Input: part model. Units: mm. Frame: model coordinates. A direction names the side the tool comes from. Coordinates: 2 decimals unless noted, no trailing zeros.
from build123d import *

# Parameters (mm, degrees)
SKETCH1_W               = 20
SKETCH1_H               = 20
SKETCH1_R               = 18.6
BOSS_EXTRUDE1_DEPTH     = 25
FILLET1_R               = 170
FILLET2_R               = 170
FILLET3_R               = 3
BOSS_EXTRUDE2_START     = -20
SKETCH2_R               = 18.6
SKETCH2_R_2             = 17.6
BOSS_EXTRUDE2_DEPTH     = 16
CHAMFER1_SIZE           = 0.5
CUT_EXTRUDE1_DEPTH      = 96
CUT_EXTRUDE1_DEPTH_BACK = 16
CUT_EXTRUDE2_START      = -8.5
SKETCH4_R               = 2.9
CUT_EXTRUDE2_DEPTH      = 46
CUT_EXTRUDE3_START      = -8
SKETCH5_R               = 1.48
CUT_EXTRUDE3_DEPTH      = 46


with BuildPart() as part:
    # Sketch1 → Boss-Extrude1 (new body)
    with BuildSketch(Plane(origin=(0, 0, 0), x_dir=(1, 0, 0), z_dir=(0, 1, 0))):
        with BuildLine():
            Line((-78.9, -20), (78.9, -20))
            Line((78.9, -20), (142.053074305, -14.2536949))
            ThreePointArc((142.053074305, -14.2536949), (167.546506822, 19.026935088), (132.290205184, 41.709717738))
            Line((132.290205184, 41.709717738), (48.9, 20))
            Line((48.9, 20), (7.809449404, 20))
            ThreePointArc((7.809449404, 20), (0, 14.05), (-7.809449404, 20))
            Line((-7.809449404, 20), (-48.9, 20))
            Line((-48.9, 20), (-132.290204174, 41.709717475))
            ThreePointArc((-132.290204174, 41.709717475), (-167.546506732, 19.026935602), (-142.053074305, -14.2536949))
            Line((-142.053074305, -14.2536949), (-78.9, -20))
        make_face()
        with Locations((-63.9, 0)):
            Rectangle(SKETCH1_W, SKETCH1_H, mode=Mode.SUBTRACT)
        with Locations((63.9, 0)):
            Rectangle(SKETCH1_W, SKETCH1_H, mode=Mode.SUBTRACT)
        with Locations(Location((139.47052489, 14.12905406, 0), (0, 0, 270))):
            Circle(SKETCH1_R, mode=Mode.SUBTRACT)
        with Locations(Location((-139.47052489, 14.12905406, 0), (0, 0, 270))):
            Circle(SKETCH1_R, mode=Mode.SUBTRACT)
    extrude(amount=BOSS_EXTRUDE1_DEPTH)

    # Fillet1
    # the kernel refuses this fillet: 170 mm, written as the material it takes off along each edge
    with BuildSketch(Plane(origin=(78.9, -19.295542523, 20), x_dir=(-1, 0, 0), z_dir=(0, 1, 0)), Plane(origin=(-78.9, -19.295542523, 20), x_dir=(-0.995885928416444, 0, -0.09061576894844221), z_dir=(0, 1, 0))) as fillet1_piece_1:
        with BuildLine():
            CenterArc((FILLET1_R * 0.045401276525, -FILLET1_R), FILLET1_R, 90, 5.199032807)
            Line((-FILLET1_R * 0.0452144924234, -FILLET1_R * 0.00411407158356), (0, 0))
            Line((0, 0), (FILLET1_R * 0.045401276525, 0))
        make_face()
    extrude(amount=63.591085046, mode=Mode.SUBTRACT)

    # Fillet2
    fillet2_edges = [part.edges().sort_by_distance(p)[0] for p in [
        (-48.9, 12.5, -20),
        (48.9, 12.5, -20),
    ]]
    fillet(fillet2_edges, radius=FILLET2_R)

    # Fillet3
    fillet3_edges = [part.edges().sort_by_distance(p)[0] for p in [
        (48.723757294, 25, -21.376513431),
        (-48.723757294, 0, -21.376513431),
        (-48.723757294, 25, -21.376513431),
        (167.546506822, 25, -19.026935088),
        (-167.546506732, 0, -19.026935602),
        (167.546506822, 0, -19.026935088),
        (-167.546506732, 25, -19.026935602),
        (114.319769009, 0, 16.777151365),
        (114.319769009, 25, 16.777151365),
        (0, 0, 20),
        (-114.319769009, 0, 16.777151365),
        (-78.892057589, 0, 19.825061948),
        (78.892057589, 0, 19.825061948),
        (0, 25, 20),
        (-114.319769009, 25, 16.777151365),
        (-78.892057589, 25, 19.825061948),
        (78.892057589, 25, 19.825061948),
        (17.471699722, 0, -20),
        (17.471699722, 25, -20),
        (101.12706922, 0, -33.596739912),
        (101.12706922, 25, -33.596739912),
        (-101.127068716, 0, -33.59673978),
        (-101.127068716, 25, -33.59673978),
        (-17.471699722, 0, -20),
        (-17.471699722, 25, -20),
        (48.723757294, 0, -21.376513431),
    ]]
    fillet(fillet3_edges, radius=FILLET3_R)

    # Sketch2 → Boss-Extrude2 (add)
    # profile 1 of 2: a face of its own
    with BuildSketch(Plane(origin=(0, 25, 0), x_dir=(1, 0, 0), z_dir=(0, 1, 0)).offset(BOSS_EXTRUDE2_START)):
        with Locations(Location((139.47052489, 14.12905406, 0), (0, 0, 270))):
            Circle(SKETCH2_R)
        with Locations(Location((139.47052489, 14.12905406, 0), (0, 0, 270))):
            Circle(SKETCH2_R_2, mode=Mode.SUBTRACT)
    # profile 2 of 2: a face of its own
    with BuildSketch(Plane(origin=(0, 25, 0), x_dir=(1, 0, 0), z_dir=(0, 1, 0)).offset(BOSS_EXTRUDE2_START)):
        with Locations(Location((-139.47052489, 14.12905406, 0), (0, 0, 270))):
            Circle(SKETCH2_R)
        with Locations(Location((-139.47052489, 14.12905406, 0), (0, 0, 270))):
            Circle(SKETCH2_R_2, mode=Mode.SUBTRACT)
    extrude(amount=BOSS_EXTRUDE2_DEPTH)

    # Chamfer1
    chamfer1_edges = [part.edges().sort_by_distance(p)[0] for p in [
        (139.47052489, 5, -31.72905406),
        (139.47052489, 21, -31.72905406),
        (-139.47052489, 5, -31.72905406),
        (-139.47052489, 21, -31.72905406),
    ]]
    chamfer(chamfer1_edges, length=CHAMFER1_SIZE)

    # Sketch3 → Cut-Extrude1 (cut, two sides: drawn at the far end of the back side and taken through both)
    with BuildSketch(Plane(origin=(0, 0, 10), x_dir=(-1, 0, 0), z_dir=(0, 0, -1)).offset(-CUT_EXTRUDE1_DEPTH_BACK)):
        with BuildLine():
            ThreePointArc((65.38, 12.5), (63.9, 13.98), (62.42, 12.5))
            Line((62.42, 12.5), (65.38, 12.5))
        make_face()
        with BuildLine():
            Line((65.38, 12.5), (62.42, 12.5))
            ThreePointArc((62.42, 12.5), (63.9, 11.02), (65.38, 12.5))
        make_face()
        with BuildLine():
            ThreePointArc((-62.42, 12.5), (-63.9, 13.98), (-65.38, 12.5))
            Line((-65.38, 12.5), (-62.42, 12.5))
        make_face()
        with BuildLine():
            Line((-62.42, 12.5), (-65.38, 12.5))
            ThreePointArc((-65.38, 12.5), (-63.9, 11.02), (-62.42, 12.5))
        make_face()
    extrude(amount=CUT_EXTRUDE1_DEPTH + CUT_EXTRUDE1_DEPTH_BACK, mode=Mode.SUBTRACT)

    # Sketch4 → Cut-Extrude2 (cut)
    with BuildSketch(Plane.XY.offset(-10).offset(CUT_EXTRUDE2_START)):
        with Locations((-63.9, 12.5)):
            Circle(SKETCH4_R)
        with Locations((63.9, 12.5)):
            Circle(SKETCH4_R)
    extrude(amount=-CUT_EXTRUDE2_DEPTH, mode=Mode.SUBTRACT)

    # Sketch5 → Cut-Extrude3 (cut)
    # profile 1 of 2: a face of its own
    with BuildSketch(Plane(origin=(0, 0, 10), x_dir=(-1, 0, 0), z_dir=(0, 0, -1)).offset(CUT_EXTRUDE3_START)):
        Polygon((65.525, 15.314582562), (62.275, 15.314582562), (60.65, 12.5), (62.275, 9.685417438), (65.525, 9.685417438), (67.15, 12.5), align=None)
        with Locations(Location((63.9, 12.5, 0), (0, 0, 180))):
            Circle(SKETCH5_R, mode=Mode.SUBTRACT)
    # profile 2 of 2: a face of its own
    with BuildSketch(Plane(origin=(0, 0, 10), x_dir=(-1, 0, 0), z_dir=(0, 0, -1)).offset(CUT_EXTRUDE3_START)):
        Polygon((-62.225, 15.401185103), (-65.575, 15.401185103), (-67.25, 12.5), (-65.575, 9.598814897), (-62.225, 9.598814897), (-60.55, 12.5), align=None)
    extrude(amount=-CUT_EXTRUDE3_DEPTH, mode=Mode.SUBTRACT)


solid = part.part
Item 1: Access query for faces 4 (the face through (157.912, 22.972, -16.55)), 5 (the face through (18, 12, -20)), 6 (the face through (157.912, 2.465, -16.55)), 7 (the face through (-100.918, 0.855, -32.61)). Directions: +Z, -Z, +X, -X, +Y, -Y. A direction counts if a zero-diameter tool reaches every point of the face in a straight line with its end or side. Return the directions, or none.
Response values:
face 4: +Y
face 5: -Z, +Y, -Y
face 6: -Y
face 7: -Z, -Y
Item 2: Draft query along Y for faces 1 (the face through (-66.8, 12.6, -21.6)), 2 (the face through (-157.3, 5, -10.1)), 3 (the face through (167.65, 12.37, -18.38)). Return one class per face: pulls with the +Y half, pulls with the -Y half, needs draft (parallel to the pull), parting line crosses it, or undercut.
Response values:
face 1: undercut
face 2: pulls with the -Y half
face 3: needs draft
Item 3: Ray query, probe 1 along X at (y, z) = (8.75, -13.5); probe 2 along X at (y, z) = (12.25, 7); probe 3 along Z at (x, y) = (-69, 5). Return the intervals inside material, ascending.
Response values:
probe 1: x = -167.96 to -157.06, -121.88 to 121.88, 157.06 to 167.96
probe 2: x = -158.6 to -73.9, -53.9 to 53.9, 73.9 to 158.6
probe 3: z = -25.24 to -10, 10 to 20
Item 4: Pin query (flat end, axial travel): pin 1 Ø4 at (x, y) = (25.5, 4.5) entering from -Z; pin 2 Ø1.6 at (x, z) = (-63.5, 19.5) entering from -Y; pin 3 Ø10 at (y, z) = (6, -25.5) entering from -X; pin 4 Ø18.5 at (x, z) = (-147.5, -13.5) entering from +Y. Return the tip coordinate at first contact, or that it passes through.
Response values:
pin 1: stops at z = -20
pin 2: stops at y = 0.53
pin 3: stops at x = -167.25
pin 4: passes through
